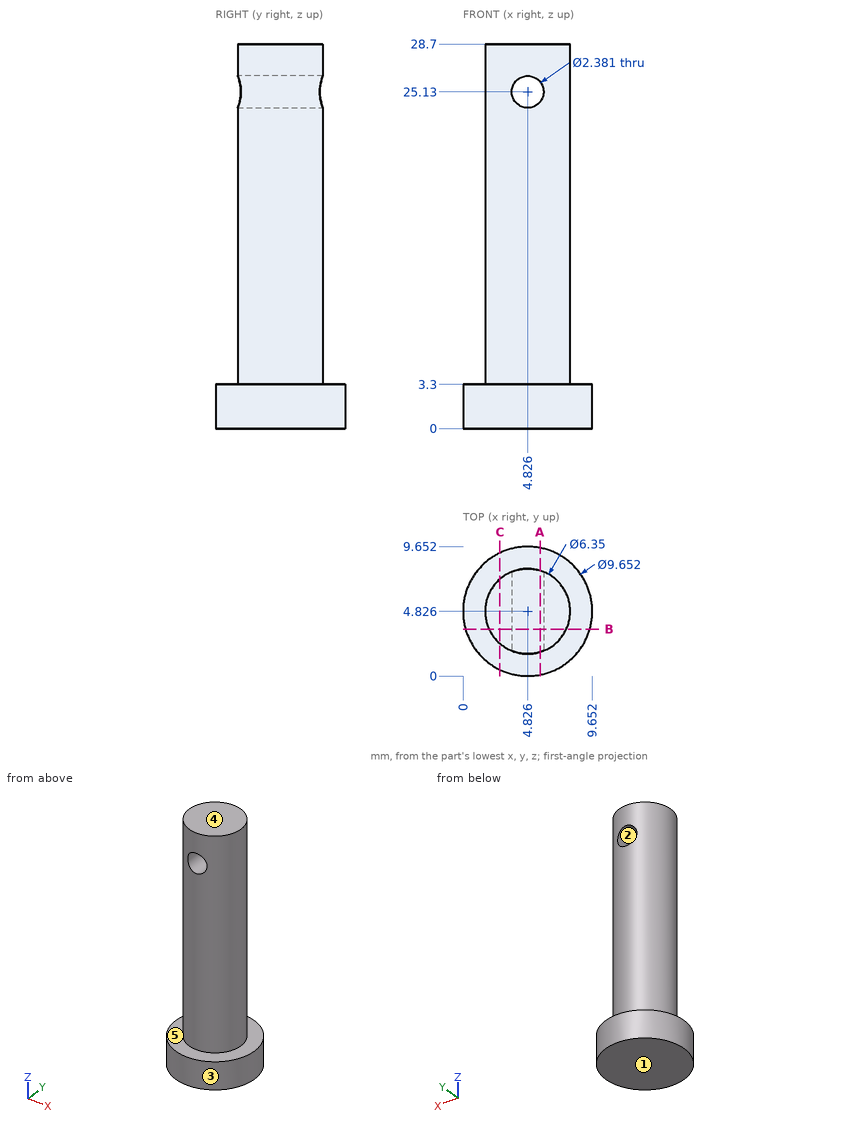
Verification items for this drawing (mm, ordinates from the low corner). A direction names the side the tool comes from. Give positions to 0.01 mm unless a question says otherwise; leave off trailing zeros. Loops run counter-clockwise (first coordinate to the right, second up) from the corner with the lowest first, then second, coordinate; pieces in that order, holes last. Notation, with made-up numbers: M 74,-31.75 L 94,-31.75 A27 cw 94,-4.75 Z; hole C 5.25,58 d4. An arc over 180 degrees is marked long. Answer as a JSON object with one key per item and string values. Group by question number.
Q1. Access from +Z, -Z, +X, -X, +Y, -Y to the whole of each face (thin tool, end or side, straight path). Record for the marked faces 4 and 5.
Q2. Material ranges on line 1 along Z through (x, y) = (5, 0.5); line 2 along Y through (x, z) = (4.75, 22.75); line 3 along X through (y, z) = (4.5, 25.13) (1 decimal), recorded low to high. Write a range as [from, to].
Q3. Cross-section at B-B on y = 3.5. Record the cut outline in (x, z), then the cut area to 3 significant figures.
Q4. Go/stop test with flat-tipped pins: P1, Ø2, axis at y = 5.5, z = 13.5, coming from the +X side; P2, Ø3, axis at x = 4.826, z = 25.13, coming from the +Y side; P3, Ø1, axis at x = 5.5, z = 19, coming from the -Y side. Record where each tip stops, or that it passes through.
Q5. Release check for a two-part mould opening along Z. For the marked faces 1, 2 and 3 record: released by +Z, released by -Z, zero draft, split by the parting line, or undercut.
Q6. Cross-section at A-A on x = 5.75. Record the cut outline in (y, z), then the cut area to 3 significant figures.
Q7. Cross-section at C-C on x = 2.75. Record the cut outline in (y, z), then the cut area to 3 significant figures.
Evaluation:
{
 "1": {"face 4": "+Z, +X, -X, +Y, -Y", "face 5": "+Z"},
 "2": {"line 1": "z = [0, 3.3]", "line 2": "y = [1.65, 8]", "line 3": "x = [1.7, 3.6], [6, 8]"},
 "3": {"outline": "M 0.19,0 L 9.47,0 L 9.47,3.3 L 7.71,3.3 L 7.71,28.7 L 1.94,28.7 L 1.94,3.3 L 0.19,3.3 Z; hole C 4.83,25.13 d2.38", "area": "173 mm2"},
 "4": {"P1": "stops at x = 8", "P2": "stops at y = 8", "P3": "stops at y = 1.66"},
 "5": {"face 1": "released by -Z", "face 2": "undercut", "face 3": "zero draft"},
 "6": {"outline": "M 0.09,0 L 9.56,0 L 9.56,3.3 L 7.86,3.3 L 7.86,24.38 L 1.79,24.38 L 1.79,3.3 L 0.09,3.3 Z; M 1.79,25.88 L 7.86,25.88 L 7.86,28.7 L 1.79,28.7 Z", "area": "176 mm2"},
 "7": {"outline": "M 0.47,0 L 9.18,0 L 9.18,3.3 L 7.23,3.3 L 7.23,28.7 L 2.42,28.7 L 2.42,3.3 L 0.47,3.3 Z", "area": "151 mm2"}
}
